Source: CAD feature listing. Evaluate the final solid. Frame: model axes, mm. A direction names the side the tool comes from. Coordinates: 2 decimals unless noted, no trailing zeros. Loops run counter-clockwise (first coordinate to the right, second up) from the corner with the lowest first, then second, coordinate; pieces in that order, holes last.
from build123d import *

# Parameters (mm, degrees)
F0_R     = 19.05
F0_R_2   = 4.056964
F1_DEPTH = 6.35
F2_SIZE  = 2.032
F3_SIZE  = 0.635


with BuildPart() as f1:
    # F0 (on Top) → F1 (new body)
    with BuildSketch(Plane.XY):
        Circle(F0_R)
        with BuildLine():
            ThreePointArc((-10.56212, -9.204333), (0, 0.146205), (10.56212, -9.204333))
            ThreePointArc((10.56212, -9.204333), (8.348809, -12.033548), (5.519595, -9.820236))
            ThreePointArc((5.519595, -9.820236), (0, -4.933795), (-5.519595, -9.820236))
            ThreePointArc((-5.519595, -9.820236), (-8.348809, -12.033548), (-10.56212, -9.204333))
        make_face(mode=Mode.SUBTRACT)
        with Locations((-8.040858, 8.613517)):
            Circle(F0_R_2, mode=Mode.SUBTRACT)
        with Locations((8.040858, 8.613517)):
            Circle(F0_R_2, mode=Mode.SUBTRACT)
    extrude(amount=F1_DEPTH)

    # F2
    f2_edges = [f1.edges().sort_by_distance(p)[0] for p in [
        (0, 0.146205, 6.35),
        (0, 0.146205, 0),
        (0, -4.933795, 6.35),
        (8.348809, -12.033548, 6.35),
        (-8.348809, -12.033548, 6.35),
        (8.348809, -12.033548, 0),
        (0, -4.933795, 0),
        (-8.348809, -12.033548, 0),
        (3.983894, 8.613517, 6.35),
        (3.983894, 8.613517, 0),
        (-12.097821, 8.613517, 0),
        (-12.097821, 8.613517, 6.35),
    ]]
    chamfer(f2_edges, length=F2_SIZE)

    # F3
    f3_edges = [f1.edges().sort_by_distance(p)[0] for p in [
        (-19.05, 0, 6.35),
        (-19.05, 0, 0),
    ]]
    chamfer(f3_edges, length=F3_SIZE)


solid = f1.part
Q1. Section A-A, the plane z = 2.5. Return the cut outline in (x, y), plus the area to 3 significant figures.
Q2. Access query for faces 1 (the conical face through (7.134, 4.529, 4.445)), 2 (the cylindrical face through (-8.29, -12.04, 3.16)). Directions: +Z, -Z, +X, -X, +Y, -Y. A direction counts if a zero-diameter tool reaches every point of the face in a straight line with its end or side. Return the directions, or none.
Q3. Line query: line 1 along X through (y, z) = (5.5, 6.25); line 2 along X through (y, z) = (5.5, 4.5); line 3 along Y through (x, z) = (-6.5, 4). Output: solid intervals per line, ascending.
Q4. Contact query for flat-ended pins moving along their axis: pin 1 Ø1.5 at (x, z) = (-12, 3) entering from +Y; pin 2 Ø1 at (y, z) = (12.5, 1) entering from +X; pin 3 Ø5 at (x, y) = (-8.04, 8.61) entering from -Z; pin 4 Ø1 at (x, z) = (-2.5, 2.5) entering from +Y. Output: stop coordinate, or through.
Q5. Section B-B, the plane x = 0. Return the cut outline in (y, z) (3 decimals), plus the area to 3 significant figures.
Q6. Draft query along X for faces 3 (the cylindrical face through (-15.12, -11.59, 3.14)), 4 (the cylindrical face through (-8.92, 4.653, 3.159)), 5 (the flat face through (0, -8, 6.35)). Return one class per face: +X half, -X half, draft (parallel to the pull), parting line (faces both ways), or undercut.
Q7. Section C-C, the plane y = -7. Count the separate pieces of the cut face and the enclosed holes in it, plus the area to 3 significant figures.
Derived:
1. outline: circle Ø38.1 at (0, 0); hole circle Ø8.11 at (-8.04, 8.61); hole (-10.56, -9.2) arc R2.54 ccw to (-5.52, -9.82) arc R5.56 cw to (5.52, -9.82) arc R2.54 ccw to (10.56, -9.2) arc R10.64 ccw to start; hole circle Ø8.11 at (8.04, 8.61)
1. area: 897 mm2
2. face 1: +Z
2. face 2: +Z, -Z
3. line 1: x = -17.68 to -13.16, -2.92 to 2.92, 13.16 to 17.68
3. line 2: x = -18.24 to -10.92, -5.16 to 5.16, 10.92 to 18.24
3. line 3: y = -17.91 to -11.53, -2.07 to 4.86, 12.37 to 17.91
4. pin 1: stops at y = 15.37
4. pin 2: stops at x = 14.8
4. pin 3: passes through
4. pin 4: stops at y = 18.94
5. outline: (-19.05, 0.635) - (-18.415, 0) - (-6.966, 0) - (-4.934, 2.032) - (-4.934, 4.318) - (-6.966, 6.35) - (-18.415, 6.35) - (-19.05, 5.715) - close; (0.146, 2.032) - (2.178, 0) - (18.415, 0) - (19.05, 0.635) - (19.05, 5.715) - (18.415, 6.35) - (2.178, 6.35) - (0.146, 4.318) - close
5. area: 201 mm2
6. face 3: parting line
6. face 4: undercut
6. face 5: draft
7. separate pieces: 3
7. enclosed holes: 0
7. area: 130 mm2
